Design review of the part built by this model. Coordinates are the model's own, in mm. A direction names the side the tool comes from. Coordinates: 2 decimals unless noted, no trailing zeros. Write each loop counter-clockwise with the first axis right and the second up, starting at its lowest first coordinate (ties: lowest second). Pieces come first, ordered by that corner, then holes.
```python
from build123d import *

# Parameters (mm, degrees)
F0_W     = 254
F0_H     = 774.7
F0_W_2   = 203.2
F0_H_2   = 596.9
F0_W_3   = 152.4
F0_H_3   = 571.5
F0_W_4   = 127
F0_H_4   = 546.1
F0_H_5   = 63.5
F1_DEPTH = 101.6
F2_DEPTH = 25.4
F3_DEPTH = 63.5
F4_R     = 50.8
F5_DEPTH = 76.2


# Not quite as in the source:
# - a feature names something its author has since deleted; it is built from what else it names


with BuildPart() as f1:
    # F0 (on Front) → F1 (new body)
    with BuildSketch(Plane.XZ):
        with Locations((0, 260.35)):
            Rectangle(F0_W, F0_H)
        with Locations((0, 298.45)):
            Rectangle(F0_W_2, F0_H_2, mode=Mode.SUBTRACT)
        with Locations((0, 298.45)):
            Rectangle(F0_W_2, F0_H_2)
        with Locations((0, 296.15)):
            Rectangle(F0_W_3, F0_H_3, mode=Mode.SUBTRACT)
        with Locations((0, 296.15)):
            Rectangle(F0_W_3, F0_H_3)
        with Locations((0, 293.85)):
            Rectangle(F0_W_4, F0_H_4, mode=Mode.SUBTRACT)
        with Locations((0, -158.75)):
            Rectangle(F0_W, F0_H_5)
    extrude(amount=-F1_DEPTH)

    # F0 (on Front) → F2 (cut)
    with BuildSketch(Plane.XZ):
        with Locations((0, 298.45)):
            Rectangle(F0_W_2, F0_H_2)
        with Locations((0, 296.15)):
            Rectangle(F0_W_3, F0_H_3, mode=Mode.SUBTRACT)
    extrude(amount=-F2_DEPTH, mode=Mode.SUBTRACT)

    # F0 (on Front) → F3 (cut)
    with BuildSketch(Plane.XZ):
        with Locations((0, 296.15)):
            Rectangle(F0_W_3, F0_H_3)
        with Locations((0, 293.85)):
            Rectangle(F0_W_4, F0_H_4, mode=Mode.SUBTRACT)
    extrude(amount=-F3_DEPTH, mode=Mode.SUBTRACT)

    # F4
    f4_edges = [f1.edges().sort_by_distance(p)[0] for p in [
        (63.5, 82.55, 566.9),
        (-63.5, 82.55, 566.9),
        (-63.5, 82.55, 20.8),
        (63.5, 82.55, 20.8),
    ]]
    fillet(f4_edges, radius=F4_R)

    # F0 (on Front) → F5 (join)
    with BuildSketch(Plane.XZ):
        with Locations((0, -158.75)):
            Rectangle(F0_W, F0_H_5)
    extrude(amount=F5_DEPTH)


solid = f1.part
```
(1) Consider section D-D (x = 109). Give the boundary of the cut face in (y, z), plus the area to 3 significant figures.
(2) Consider section C-C (z = 317). Give the boundary of the cut face in (x, y).
(3) Consider section B-B (x = -31.5). Give the boundary of the cut face in (y, z).
(4) Consider section A-A (y = 86). Give the boundary of the cut face in (x, z), plus the area to 3 significant figures.
(5) Insertion check: pin 1 Ø6 at (x, z) = (54.5, -53.5) entering from -Y. The pin has a flat end and moves straight along its axis. Give the tip position at first contact, or say it passes through.
(6) Mouldability with a two-part tool opening along Z and no side actions: class faces 1 (the flat face through (-127, 53, 223)), 2 (the flat face through (-2, 14, -190.5)), 3 (the flat face through (-83, 25.4, 344)) as +Z half, -Z half, draft (parallel to the pull), parting line (faces both ways), or undercut.
(7) Wall thickness on line 1 (X direction, y = 57.5, z = 426.5); line 2 (Z direction, x = 16, y = 49.5); line 3 (X direction, y = 79.5, z = 515): over which ranges is each line inside the solid? List them lowest first.
(8) For faces 4 (the flat face through (127, 53, 223)), 5 (the cylindrical face through (48.224, 82.817, 35.286)), 6 (the flat face through (-101.6, 13, 294)), list the 3-axis set-ups (+Z, -Z, +X, -X, +Y, -Y) from which the entire face can be reached by the end or side of a thin tool; tool diameter is ignored.
Results:
1. outline: (-76.2, -190.5) - (101.6, -190.5) - (101.6, 647.7) - (0, 647.7) - (0, -127) - (-76.2, -127) - close
1. area: 90,000 mm2
2. outline: (-127, 0) - (-101.6, 0) - (-101.6, 25.4) - (-76.2, 25.4) - (-76.2, 63.5) - (-63.5, 63.5) - (-63.5, 101.6) - (-127, 101.6) - close; (63.5, 63.5) - (76.2, 63.5) - (76.2, 25.4) - (101.6, 25.4) - (101.6, 0) - (127, 0) - (127, 101.6) - (63.5, 101.6) - close
3. outline: (-76.2, -190.5) - (101.6, -190.5) - (101.6, 24.41) - (63.5, 24.41) - (63.5, 10.4) - (25.4, 10.4) - (25.4, 0) - (0, 0) - (0, -127) - (-76.2, -127) - close; (0, 596.9) - (25.4, 596.9) - (25.4, 581.9) - (63.5, 581.9) - (63.5, 563.29) - (101.6, 563.29) - (101.6, 647.7) - (0, 647.7) - close
4. outline: (-127, -190.5) - (127, -190.5) - (127, 647.7) - (-127, 647.7) - close; hole (-63.5, 71.6) arc R50.8 ccw to (-12.7, 20.8) - (12.7, 20.8) arc R50.8 ccw to (63.5, 71.6) - (63.5, 516.1) arc R50.8 ccw to (12.7, 566.9) - (-12.7, 566.9) arc R50.8 ccw to (-63.5, 516.1) - close
4. area: 146,000 mm2
5. pin 1: stops at y = 0
6. face 1: draft
6. face 2: -Z half
6. face 3: undercut
7. line 1: x = -127 to -76.2, 76.2 to 127
7. line 2: z = -190.5 to 10.4, 581.9 to 647.7
7. line 3: x = -127 to -63.5, 63.5 to 127
8. face 4: +Z, -Z, +X, +Y, -Y
8. face 5: +Y, -Y
8. face 6: -Y
